from build123d import *

# Parameters (mm, degrees)
BOSS_EXTRUDE1_DEPTH = 20
SKETCH2_R           = 10
BOSS_EXTRUDE2_DEPTH = 80
SKETCH3_R           = 12.5
BOSS_EXTRUDE3_DEPTH = 40


with BuildPart() as part:
    # Sketch1 → Boss-Extrude1 (new body)
    with BuildSketch(Plane.XY):
        with BuildLine():
            Line((-40.373207368, -5), (-5, -5))
            Line((-5, -5), (-5, -40.373207368))
            ThreePointArc((-5, -40.373207368), (0, -45.373207368), (5, -40.373207368))
            Line((5, -40.373207368), (5, -5))
            Line((5, -5), (40.373207368, -5))
            ThreePointArc((40.373207368, -5), (45.373207368, 0), (40.373207368, 5))
            Line((40.373207368, 5), (5, 5))
            Line((5, 5), (5, 40.373207368))
            ThreePointArc((5, 40.373207368), (0, 45.373207368), (-5, 40.373207368))
            Line((-5, 40.373207368), (-5, 5))
            Line((-5, 5), (-40.373207368, 5))
            ThreePointArc((-40.373207368, 5), (-45.373207368, 0), (-40.373207368, -5))
        make_face()
    extrude(amount=BOSS_EXTRUDE1_DEPTH)

    # Sketch2 → Boss-Extrude2 (add)
    with BuildSketch(Plane.XY.offset(20)):
        Circle(SKETCH2_R)
    extrude(amount=-BOSS_EXTRUDE2_DEPTH)

    # Sketch3 → Boss-Extrude3 (add)
    with BuildSketch(Plane.XY.offset(20)):
        Circle(SKETCH3_R)
    extrude(amount=-BOSS_EXTRUDE3_DEPTH)


solid = part.part
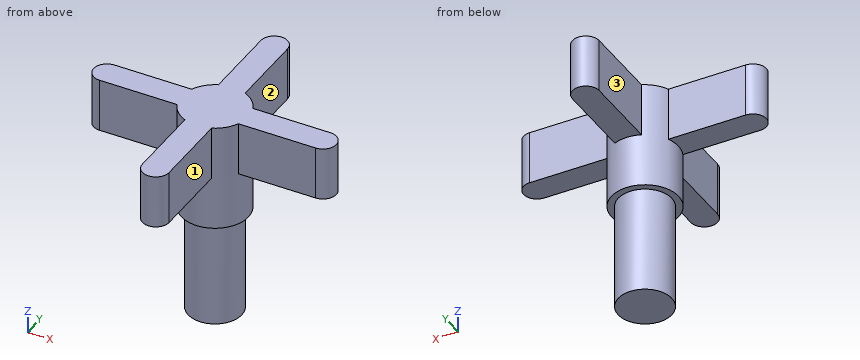
Part model, mm, in its own coordinate system. Face numbers are marked on the shaded views. A direction names the side the tool comes from. Coordinates: 2 decimals unless noted, no trailing zeros. Write each loop counter-clockwise with the first axis right and the second up, starting at its lowest first coordinate (ties: lowest second). Pieces come first, ordered by that corner, then holes. Notation, with made-up numbers: M -13.5,55.25 L -1.5,55.25 A36 ccw -1.5,91.25 Z; hole C 53,20 d1. An arc over 180 degrees is marked long. Return JSON: item names as keys, results as strings.
1. 3-axis set-ups, long thin cutter, end or side, ignore diameter. For the marked faces 1, 2 and 3: which of +Z, -Z, +X, -X, +Y, -Y reach the whole face in a straight line?
Determined:
{"face 1": "+Z, -Z, +X, -Y", "face 2": "+Z, -Z, +X, +Y", "face 3": "+Z, -Z, -X, +Y"}
2. Flat gauge pins, fed straight in: pin 1 Ø6 at (x, z) = (26, 9) entering from -Y; pin 2 Ø6 at (y, z) = (14, -41) entering from -X; pin 3 Ø10 at (y, z) = (-30.5, 8.5) entering from -X; pin 4 Ø10 at (x, y) = (-15.5, -9) entering from -Z. Where does each tip first touch, or does it go through?
Determined:
{"pin 1": "y = -5", "pin 2": "through", "pin 3": "x = -5", "pin 4": "z = 0"}
3. Saw through at A-A, the plane z = 5. Write the cut outline in (x, y), then the cut area to 3 significant figures.
Determined:
{"outline": "M -40.37,-5 L -11.46,-5 A12.5 ccw -5,-11.46 L -5,-40.37 A5 ccw 5,-40.37 L 5,-11.46 A12.5 ccw 11.46,-5 L 40.37,-5 A5 ccw 40.37,5 L 11.46,5 A12.5 ccw 5,11.46 L 5,40.37 A5 ccw -5,40.37 L -5,11.46 A12.5 ccw -11.46,5 L -40.37,5 A5 ccw Z", "area": "1,780 mm²"}
4. Probe L1, parallel to Y at x = 24, z = 3.5; L2, parallel to Z at x = 3.5, y = -22. List the from-to ranges inside material, lowest first.
Determined:
{"L1": "-5 to 5", "L2": "0 to 20"}
5. Saw through at B-B, the plane y = 0. Write the cut outline in (x, z), then the cut area to 3 significant figures.
Determined:
{"outline": "M -45.37,0 L -12.5,0 L -12.5,-20 L -10,-20 L -10,-60 L 10,-60 L 10,-20 L 12.5,-20 L 12.5,0 L 45.37,0 L 45.37,20 L -45.37,20 Z", "area": "3,110 mm²"}
6. Saw through at D-D, the plane z = -30.5. Write the cut outline in (x, y), then the cut area to 3 significant figures.
Determined:
{"outline": "C 0,0 d20", "area": "314 mm²"}
